Verification items for the finished model (mm, model axes). Face numbers are marked on the shaded views. A direction names the side the tool comes from. Round coordinates to 2 decimals unless told otherwise and drop trailing zeros. Write each loop counter-clockwise with the first axis right and the second up, starting at its lowest first coordinate (ties: lowest second). Pieces come first, ordered by that corner, then holes. Notation, with made-up numbers: (36, -16.5) - (88, -16.5) arc R16 cw to (88, -2.5) - close; hole circle Ø9 at (2, 82.25). An arc over 180 degrees is marked (long way). Answer as a JSON object with one key per item and string values.
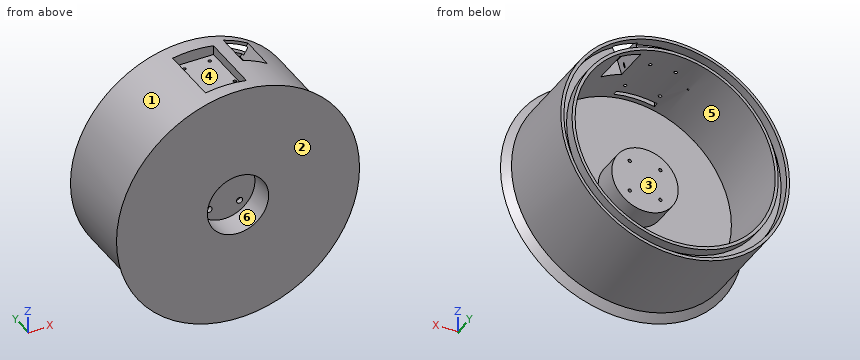
```python
from build123d import *

# Parameters (mm, degrees)
SKETCH1_R               = 112
BOSS_EXTRUDE3_DEPTH     = 90
SKETCH9_R               = 109
SKETCH9_R_2             = 101
CUT_EXTRUDE6_DEPTH      = 10
SKETCH4_W               = 40
SKETCH4_H               = 60
CUT_EXTRUDE2_DEPTH      = 26
CUT_EXTRUDE2_DEPTH_BACK = 4
SKETCH12_R              = 112
BOSS_EXTRUDE4_DEPTH     = 7
BOSS_EXTRUDE4_TAPER     = -45
SKETCH13_R              = 98
CUT_EXTRUDE8_DEPTH      = 80
SKETCH14_R              = 0.75
CUT_EXTRUDE9_DEPTH      = 15
SKETCH18_R              = 32.5
BOSS_EXTRUDE5_DEPTH     = 25
SKETCH16_R              = 1.6
CUT_EXTRUDE11_DEPTH     = 98.0000001
SKETCH17_R              = 3
CUT_EXTRUDE12_DEPTH     = 30
SKETCH19_R              = 30
CUT_EXTRUDE13_DEPTH     = 25
SKETCH20_W              = 40
SKETCH20_H              = 5
CUT_EXTRUDE14_DEPTH     = 25
SKETCH21_R              = 1.55
CUT_EXTRUDE15_DEPTH     = 25
CUT_EXTRUDE16_DEPTH     = 35


with BuildPart() as part:
    # Sketch1 → Boss-Extrude3 (new body)
    with BuildSketch(Plane(origin=(0, 0, 0), x_dir=(1, 0, 0), z_dir=(0, 1, 0))):
        Circle(SKETCH1_R)
    extrude(amount=BOSS_EXTRUDE3_DEPTH)

    # Sketch9 → Cut-Extrude6 (cut)
    with BuildSketch(Plane(origin=(0, 90, 0), x_dir=(1, 0, 0), z_dir=(0, 1, 0))):
        Circle(SKETCH9_R)
        Circle(SKETCH9_R_2, mode=Mode.SUBTRACT)
    extrude(amount=-CUT_EXTRUDE6_DEPTH, mode=Mode.SUBTRACT)

    # Sketch4 → Cut-Extrude2 (cut, two sides)
    with BuildSketch(Plane.XY.offset(105)) as cut_extrude2_sk:
        with Locations((0, 45)):
            Rectangle(SKETCH4_W, SKETCH4_H)
    extrude(amount=CUT_EXTRUDE2_DEPTH, mode=Mode.SUBTRACT)
    extrude(cut_extrude2_sk.sketch, amount=-CUT_EXTRUDE2_DEPTH_BACK, mode=Mode.SUBTRACT)

    # Sketch12 → Boss-Extrude4 (add)
    with BuildSketch(Plane.XZ):
        Circle(SKETCH12_R)
    extrude(amount=BOSS_EXTRUDE4_DEPTH, taper=BOSS_EXTRUDE4_TAPER)

    # Sketch13 → Cut-Extrude8 (cut)
    with BuildSketch(Plane(origin=(0, 90, 0), x_dir=(1, 0, 0), z_dir=(0, 1, 0))):
        Circle(SKETCH13_R)
    extrude(amount=-CUT_EXTRUDE8_DEPTH, mode=Mode.SUBTRACT)

    # Sketch14 → Cut-Extrude9 (cut)
    with BuildSketch(Plane.XY.offset(101)):
        with Locations((-31.25, 55.25)):
            Circle(SKETCH14_R)
        with Locations((31.25, 55.25)):
            Circle(SKETCH14_R)
        with Locations((31.25, 7.75)):
            Circle(SKETCH14_R)
        with Locations((-31.25, 7.75)):
            Circle(SKETCH14_R)
    extrude(amount=-CUT_EXTRUDE9_DEPTH, mode=Mode.SUBTRACT)

    # Sketch18 → Boss-Extrude5 (add)
    with BuildSketch(Plane(origin=(0, 10, 0), x_dir=(1, 0, 0), z_dir=(0, 1, 0))):
        Circle(SKETCH18_R)
    extrude(amount=BOSS_EXTRUDE5_DEPTH)

    # Sketch16 → Cut-Extrude11 (cut, through all)
    with BuildSketch(Plane.XZ.offset(7)):
        with Locations((-15, 15.5)):
            Circle(SKETCH16_R)
        with Locations((15, 15.5)):
            Circle(SKETCH16_R)
        with Locations((15, -15.5)):
            Circle(SKETCH16_R)
        with Locations((-15, -15.5)):
            Circle(SKETCH16_R)
    extrude(amount=-CUT_EXTRUDE11_DEPTH, mode=Mode.SUBTRACT)

    # Sketch17 → Cut-Extrude12 (cut)
    with BuildSketch(Plane.XZ.offset(7)):
        with Locations((-15, 15.5)):
            Circle(SKETCH17_R)
        with Locations((15, 15.5)):
            Circle(SKETCH17_R)
        with Locations((-15, -15.5)):
            Circle(SKETCH17_R)
        with Locations((15, -15.5)):
            Circle(SKETCH17_R)
    extrude(amount=-CUT_EXTRUDE12_DEPTH, mode=Mode.SUBTRACT)

    # Sketch19 → Cut-Extrude13 (cut)
    with BuildSketch(Plane.XZ.offset(7)):
        Circle(SKETCH19_R)
    extrude(amount=-CUT_EXTRUDE13_DEPTH, mode=Mode.SUBTRACT)

    # Sketch20 → Cut-Extrude14 (cut)
    with BuildSketch(Plane.XY.offset(101)):
        with Locations((0, 17.5)):
            Rectangle(SKETCH20_W, SKETCH20_H)
    extrude(amount=-CUT_EXTRUDE14_DEPTH, mode=Mode.SUBTRACT)

    # Sketch21 → Cut-Extrude15 (cut)
    with BuildSketch(Plane.XY.offset(101)):
        with Locations((12.45, 67.8)):
            Circle(SKETCH21_R)
        with Locations((-12.45, 67.8)):
            Circle(SKETCH21_R)
        with Locations((-17.05, 30.54)):
            Circle(SKETCH21_R)
        with Locations((17.05, 30.54)):
            Circle(SKETCH21_R)
    extrude(amount=-CUT_EXTRUDE15_DEPTH, mode=Mode.SUBTRACT)

    # Sketch22 → Cut-Extrude16 (cut)
    with BuildSketch(Plane(origin=(22.204096953, 47.794122581, -296.404157649), x_dir=(1, 0, 0), z_dir=(0, 1, 0))):
        Polygon((-8.101888311, -337.261049447), (12.404969277, -405.762485644), (37.058002756, -394.3841625), (-1.388931435, -334.195344764), align=None)
    extrude(amount=CUT_EXTRUDE16_DEPTH, mode=Mode.SUBTRACT)


solid = part.part
```
Q1. Material ranges on line 1 along Y through (x, z) = (17.05, 97.6); line 2 along Y through (x, z) = (31, 97); line 3 along Z through (x, y) = (22.5, 12), recorded low to high. Write a range as [from, to].
Geometry check:
{"line 1": "y = [-7, 15], [20, 28.99], [32.09, 90]", "line 2": "y = [-7, 7.04], [8.46, 47.79]", "line 3": "z = [-109.72, -95.38], [-23.45, -19.84], [19.84, 23.45], [95.38, 109.72]"}
Q2. Release check for a two-part mould opening along Z. For the marked faces 1, 2 and 3 record: released by +Z, released by -Z, zero draft, split by the parting line, or undercut.
Geometry check:
{"face 1": "split by the parting line", "face 2": "zero draft", "face 3": "undercut"}
Q3. Gauge pin test, flat ends, axial feed: P1, Ø5, axis at x = 15, z = 16.5, coming from the -Y side; P2, Ø9.5, axis at x = -15, z = -15.5, coming from the +Y side; P3, Ø3, axis at y = 12.5, z = -64.5, coming from the +X side. Record the tip position at first contact, or that the pin passes through.
Geometry check:
{"P1": "stops at y = 18", "P2": "stops at y = 35", "P3": "stops at x = 92.6"}
Q4. Section check A-A, the plane y = 26. Record the cut outline in (x, z), then the cut area to 3 significant figures.
Geometry check:
{"outline": "circle Ø65 at (0, 0); (-20, 101) - (-20, 110.2) arc R112 ccw (long way) to (20, 110.2) - (20, 101) - close; hole circle Ø196 at (0, 0); hole circle Ø3.2 at (-15, -15.5); hole circle Ø3.2 at (-15, 15.5); hole circle Ø3.2 at (15, -15.5); hole circle Ø3.2 at (15, 15.5)", "area": "12,100 mm2"}
Q5. Section check B-B, the plane y = 42.5. Record the cut outline in (x, z), then the cut area to 3 significant figures.
Geometry check:
{"outline": "(-20, 101) - (-20, 110.2) arc R112 ccw (long way) to (20, 110.2) - (20, 101) - close; hole circle Ø196 at (0, 0)", "area": "8,820 mm2"}
Q6. Set-up check for the marked faces 4, 5 and 6: record each of +Z, -Z, +X, -X, +Y, -Y from which the full face is reachable in a straight line by a thin tool's end or side.
Geometry check:
{"face 4": "+Z", "face 5": "+Y", "face 6": "-Y"}
